Input: part model. Units: mm. Frame: model coordinates. A direction names the side the tool comes from. Coordinates: 2 decimals unless noted, no trailing zeros. Write each loop counter-clockwise with the first axis right and the second up, starting at its lowest first coordinate (ties: lowest second). Pieces come first, ordered by that corner, then holes.
from build123d import *

# Parameters (mm, degrees)
SKETCH2_R           = 3.048
BOSS_EXTRUDE1_DEPTH = 3.81
SKETCH3_R           = 3.556
BOSS_EXTRUDE2_DEPTH = 1.27
SKETCH4_W           = 3.556
SKETCH4_H           = 3.556
CUT_EXTRUDE1_DEPTH  = 6.08


with BuildPart() as part:
    # Sketch2 → Boss-Extrude1 (new body)
    with BuildSketch(Plane(origin=(0, 0, 0), x_dir=(0, 0, -1), z_dir=(1, 0, 0))):
        Circle(SKETCH2_R)
    extrude(amount=BOSS_EXTRUDE1_DEPTH)

    # Sketch3 → Boss-Extrude2 (add)
    with BuildSketch(Plane(origin=(3.81, 0, 0), x_dir=(0, 0, -1), z_dir=(1, 0, 0))):
        Circle(SKETCH3_R)
    extrude(amount=BOSS_EXTRUDE2_DEPTH)

    # Sketch4 → Cut-Extrude1 (cut, through all)
    with BuildSketch(Plane.ZY):
        Rectangle(SKETCH4_W, SKETCH4_H)
    extrude(amount=-CUT_EXTRUDE1_DEPTH, mode=Mode.SUBTRACT)


solid = part.part
Item 1: Pin query (flat end, axial travel): pin 1 Ø1 at (x, z) = (4, -1) entering from +Y; pin 2 Ø3 at (x, z) = (1, -1) entering from +Y; pin 3 Ø2 at (x, z) = (1.5, 3) entering from +Y. Return the tip coordinate at first contact, or that it passes through.
Item 2: Access query for faces 1 (the face through (5.08, -2, 0)), 2 (the face through (3, 0, -1.778)), 3 (the face through (1.88, 3.02, 0.4)). Directions: +Z, -Z, +X, -X, +Y, -Y. A direction counts if a zero-diameter tool reaches every point of the face in a straight line with its end or side. Return the directions, or none.
Item 3: Section query D-D, the plane x = 3.5. Return loops of the section in (y, z), then the cut area to 3 significant figures.
Item 4: Material intervals for line 1 (Y direction, x = 1.9, z = 0); line 2 (Z direction, x = 0.25, y = -1.5); line 3 (Z direction, x = 4.05, y = -1.5), sorted ascending.
Item 5: Pull-direction query (Z, two-part tool) for faces 4 (the face through (3, 1.778, 0)), 5 (the face through (3, -1.778, 0)), 6 (the face through (0, -2, 0)), 7 (the face through (4.44, -3.47, 0.77)); classes: released by +Z, released by -Z, zero draft, split by the parting line, or undercut.
Item 6: Section query A-A, the plane z = 0. Return loops of the section in (x, y), then the cut area to 3 significant figures.
Item 7: Section query C-C, the plane x = 4.65. Return loops of the section in (y, z).
The answers:
1. pin 1: stops at y = 3.52
1. pin 2: stops at y = 3.05
1. pin 3: stops at y = 2.3
2. face 1: +Z, -Z, +X, +Y, -Y
2. face 2: +X, -X
2. face 3: -X
3. outline: circle Ø6.1 at (0, 0); hole (-1.78, -1.78) - (1.78, -1.78) - (1.78, 1.78) - (-1.78, 1.78) - close
3. area: 16.5 mm2
4. line 1: y = -3.05 to -1.78, 1.78 to 3.05
4. line 2: z = -2.65 to -1.78, 1.78 to 2.65
4. line 3: z = -3.22 to -1.78, 1.78 to 3.22
5. face 4: undercut
5. face 5: undercut
5. face 6: zero draft
5. face 7: split by the parting line
6. outline: (0, -3.05) - (3.81, -3.05) - (3.81, -3.56) - (5.08, -3.56) - (5.08, -1.78) - (0, -1.78) - close; (0, 1.78) - (5.08, 1.78) - (5.08, 3.56) - (3.81, 3.56) - (3.81, 3.05) - (0, 3.05) - close
6. area: 14.2 mm2
7. outline: circle Ø7.11 at (0, 0); hole (-1.78, -1.78) - (1.78, -1.78) - (1.78, 1.78) - (-1.78, 1.78) - close
